```python
from build123d import *

# Parameters (mm, degrees)
EXTRUDE_THIN1_DEPTH = 85
BOSS_EXTRUDE1_DEPTH = 15
BOSS_EXTRUDE2_DEPTH = 16
FILLET1_R           = 21
BOSS_EXTRUDE3_DEPTH = 15
FILLET2_R           = 16
SKETCH6_R           = 12
CUT_EXTRUDE2_DEPTH  = 272.746205125
FILLET3_R           = 30
SKETCH7_R           = 12
CUT_EXTRUDE3_DEPTH  = 281.766807155
SKETCH9_R           = 10
CUT_EXTRUDE4_DEPTH  = 287.609490422


with BuildPart() as part:
    # Sketch1 → Extrude-Thin1 (new body)
    with BuildSketch(Plane.XY):
        Polygon((0, 0), (150, 0), (150, 28), (235, 28), (235, 43), (135, 43), (135, 15), (0, 15), align=None)
    extrude(amount=-EXTRUDE_THIN1_DEPTH)

    # Sketch2 → Boss-Extrude1 (add)
    with BuildSketch(Plane.ZY):
        Polygon((0, 15), (0, 118), (-112, 118), (-112, 76), (-43, 76), (-43, 15), align=None)
    extrude(amount=-BOSS_EXTRUDE1_DEPTH)

    # Sketch3 → Boss-Extrude2 (add)
    with BuildSketch(Plane.ZY.offset(-135)):
        with BuildLine():
            Line((0, 43), (-79.111854281, 112.751806515))
            ThreePointArc((-79.111854281, 112.751806515), (-106.449245092, 113.128168106), (-110.990788091, 86.168031394))
            Line((-110.990788091, 86.168031394), (-85, 43))
            Line((-85, 43), (0, 43))
        make_face()
    extrude(amount=-BOSS_EXTRUDE2_DEPTH)

    # Fillet1
    fillet1_edges = [part.edges().sort_by_distance(p)[0] for p in [
        (7.5, 76, -112),
        (7.5, 118, -112),
        (7.5, 118, 0),
    ]]
    fillet(fillet1_edges, radius=FILLET1_R - 0.0001)  # a hair under: the kernel refuses the full size

    # Sketch5 → Boss-Extrude3 (add)
    with BuildSketch(Plane(origin=(0, 43, 0), x_dir=(1, 0, 0), z_dir=(0, 1, 0))):
        with BuildLine():
            Line((175, 0), (235, 0))
            ThreePointArc((235, 0), (205, -30), (175, 0))
        make_face()
    extrude(amount=-BOSS_EXTRUDE3_DEPTH)

    # Fillet2
    fillet2_edges = [part.edges().sort_by_distance(p)[0] for p in [
        (175, 35.5, 0),
    ]]
    fillet(fillet2_edges, radius=FILLET2_R)

    # Sketch6 → Cut-Extrude2 (cut, through all)
    with BuildSketch(Plane(origin=(0, 43, 0), x_dir=(1, 0, 0), z_dir=(0, 1, 0))):
        with Locations(Location((205, -12, 0), (0, 0, 270))):
            Circle(SKETCH6_R)
        with Locations(Location((205, 58, 0), (0, 0, 270))):
            Circle(SKETCH6_R)
    extrude(amount=-CUT_EXTRUDE2_DEPTH, mode=Mode.SUBTRACT)

    # Fillet3
    fillet3_edges = [part.edges().sort_by_distance(p)[0] for p in [
        (235, 35.5, -85),
    ]]
    fillet(fillet3_edges, radius=FILLET3_R)

    # Sketch7 → Cut-Extrude3 (cut, through all)
    with BuildSketch(Plane(origin=(0, 15, 0), x_dir=(1, 0, 0), z_dir=(0, 1, 0))):
        with Locations(Location((75, 42, 0), (0, 0, 270))):
            Circle(SKETCH7_R)
    extrude(amount=-CUT_EXTRUDE3_DEPTH, mode=Mode.SUBTRACT)

    # Sketch9 → Cut-Extrude4 (cut, through all)
    with BuildSketch(Plane.ZY):
        with Locations((-91, 97)):
            Circle(SKETCH9_R)
        with Locations((-21, 97)):
            Circle(SKETCH9_R)
    extrude(amount=-CUT_EXTRUDE4_DEPTH, mode=Mode.SUBTRACT)


solid = part.part
```
The listing builds one solid part. Answer for the finished solid, in the listing's coordinates (mm). A direction names the side the tool comes from. Coordinates: 2 decimals unless noted, no trailing zeros. Order: outer loops, then holes, each group sorted by start corner. A loop starts at its lowest first (then second) coordinate and runs counter-clockwise, first axis right, second up. Notation, with made-up numbers: M -0.5,-28.5 L 4.5,-28.5 A8 ccw 4.5,-17.5 Z; hole C -31,49 d8. An arc over 180 degrees is marked long. Answer as a JSON object with one key per item and string values. Group by question number.
1. Section D-D on y = 52.5 is taken. Write down the section's boundary in (x, z).
2. Section A-A on y = 12 is taken. Write down the section's boundary in (x, z).
3. Section C-C on x = 78 is taken. Write down the section's boundary in (y, z), then the cut area to 3 significant figures.
4. Section B-B on z = -65 is taken. Write down the section's boundary in (x, y), then the cut area to 3 significant figures.
5. Straight lines are drawn through the part: line 1 (X direction, y = 33, z = -7.5); line 2 (Y direction, x = 205, z = -78); line 3 (X direction, y = 48.5, z = -36). For each, find the intervals that lie inside material, in ascending order.
6. A tool of negligible diameter and unlimited length cuts with its end or side. For faces 4 (the flat face through (101, 12, -85)), 5 (the flat face through (194, 43, -28)), 6 (the flat face through (193, 28, -28)), 7 (the flat face through (57, 12, 0)), from which of +Z, -Z, +X, -X, +Y, -Y can it reach the whole face along a straight path? Write none if from no direction.
7. Flat-ended cylindrical pins translate along their axes: P1, Ø1.5, axis at x = 169, z = -13, coming from the +Y side; P2, Ø10, axis at y = 76.5, z = -50, coming from the +X side; P3, Ø8, axis at y = 23, z = -46, coming from the +X side. Find the tip coordinate at first contact, or state that the pin passes through.
8. Determine the mould class of faces 1 (the flat face through (142.89, 64.89, -98.18)), 2 (the flat face through (7, 46, -43)), 3 (the cylindrical face through (216.9, 35.61, 10.44)) for opening direction Y: released by +Y, released by -Y, zero draft, split by the parting line, or undercut.
Values follow:
{
 "1": {"outline": "M 0,-43 L 15,-43 L 15,0 L 0,0 Z; M 135,-90.72 L 151,-90.72 L 151,-10.77 L 135,-10.77 Z"},
 "2": {"outline": "M 0,-85 L 150,-85 L 150,0 L 0,0 Z; hole C 75,-42 d24"},
 "3": {"outline": "M 0,-85 L 15,-85 L 15,-53.62 L 0,-53.62 Z; M 0,-30.38 L 15,-30.38 L 15,0 L 0,0 Z", "area": "926 mm2"},
 "4": {"outline": "M 0,0 L 150,0 L 150,28 L 195.25,28 L 195.25,43 L 151,43 L 151,100.31 L 135,100.31 L 135,15 L 0,15 Z; M 0,76 L 15,76 L 15,118 L 0,118 Z; M 214.75,28 L 233.28,28 L 233.28,43 L 214.75,43 Z", "area": "5,170 mm2"},
 "5": {"line 1": "0 to 15, 135 to 235", "line 2": "28 to 43", "line 3": "0 to 15, 135 to 151"},
 "6": {"face 4": "-Z, +X, -X, -Y", "face 5": "+Z, -Z, +X, +Y", "face 6": "+Z, -Z, +X, -Y", "face 7": "+Z, -X, +Y, -Y"},
 "7": {"P1": "y = 43", "P2": "x = 151", "P3": "x = 150"},
 "8": {"face 1": "released by -Y", "face 2": "undercut", "face 3": "zero draft"}
}
